The listing builds one solid part. Answer for the finished solid, in the listing's coordinates (mm). A direction names the side the tool comes from. Round coordinates to 2 decimals unless told otherwise and drop trailing zeros. Loops run counter-clockwise (first coordinate to the right, second up) from the corner with the lowest first, then second, coordinate; pieces in that order, holes last. Notation, with made-up numbers: M 67,-18.5 L 104,-18.5 A11 ccw 104,-10.5 Z; hole C 70.25,31.25 d8. An arc over 180 degrees is marked long. Answer as a JSON object with one key per item and string values.
```python
from build123d import *

# Parameters (mm, degrees)
SKETCH1_W           = 20
SKETCH1_H           = 42
BOSS_EXTRUDE1_DEPTH = 7.6
CUT_EXTRUDE1_DEPTH  = 4
THICKEN1_START      = -10
THICKEN1_DEPTH      = 20
SKETCH7_W           = 16
SKETCH7_H           = 1.6
CUT_EXTRUDE6_DEPTH  = 15


# Read off the part's stored shape, not the designer's step: Thicken1
with BuildPart() as part:
    # Sketch1 → Boss-Extrude1 (new body)
    with BuildSketch(Plane(origin=(0, 0, 0), x_dir=(1, 0, 0), z_dir=(0, 1, 0))):
        Rectangle(SKETCH1_W, SKETCH1_H)
    extrude(amount=BOSS_EXTRUDE1_DEPTH)

    # Sketch2 → Cut-Extrude1 (cut)
    with BuildSketch(Plane.XZ):
        with BuildLine():
            Line((-3.5, -17.5), (3.5, -17.5))
            Line((3.5, -17.5), (3.5, -5.5))
            ThreePointArc((3.5, -5.5), (4.085786438, -4.085786438), (5.5, -3.5))
            Line((5.5, -3.5), (8.5, -3.5))
            Line((8.5, -3.5), (8.5, 0.5))
            Line((8.5, 0.5), (5.5, 0.5))
            ThreePointArc((5.5, 0.5), (4.085786438, 1.085786438), (3.5, 2.5))
            Line((3.5, 2.5), (3.5, 17.5))
            Line((3.5, 17.5), (-3.5, 17.5))
            Line((-3.5, 17.5), (-3.5, 2.5))
            ThreePointArc((-3.5, 2.5), (-4.085786438, 1.085786438), (-5.5, 0.5))
            Line((-5.5, 0.5), (-8.5, 0.5))
            Line((-8.5, 0.5), (-8.5, -3.5))
            Line((-8.5, -3.5), (-5.5, -3.5))
            ThreePointArc((-5.5, -3.5), (-4.085786438, -4.085786438), (-3.5, -5.5))
            Line((-3.5, -5.5), (-3.5, -17.5))
        make_face()
    extrude(amount=-CUT_EXTRUDE1_DEPTH, mode=Mode.SUBTRACT)

    # Thicken1 outline → Thicken1 (add)
    with BuildSketch(Plane.YZ.offset(THICKEN1_START)):
        Polygon((0, -23), (9.6, -23), (9.6, 23), (0, 23), (0, 21), (7.6, 21), (7.6, -21), (0, -21), align=None)
    extrude(amount=THICKEN1_DEPTH)

    # Sketch7 → Cut-Extrude6 (cut)
    with BuildSketch(Plane(origin=(0, 0, -23), x_dir=(-1, 0, 0), z_dir=(0, 0, -1))):
        with Locations((0, 7.2)):
            Rectangle(SKETCH7_W, SKETCH7_H)
    extrude(amount=-CUT_EXTRUDE6_DEPTH, mode=Mode.SUBTRACT)


solid = part.part
```
Item 1: The part is cut by section C-C (z = -3). Give the vertices of the cut face in (x, y), then the cut area to 3 significant figures.
Values follow:
{"outline": "M -10,0 L -8.5,0 L -8.5,4 L 8.5,4 L 8.5,0 L 10,0 L 10,9.6 L -10,9.6 Z", "area": "124 mm^2"}
Item 2: Straight lines are drawn through the part: line 1 (Y direction, x = 2.5, z = -11); line 2 (Z direction, x = -0.25, y = 3.5); line 3 (X direction, y = 3.75, z = -12). For each, find the intervals that lie inside material, in ascending order.
Values follow:
{"line 1": "4 to 6.4, 8 to 9.6", "line 2": "-23 to -17.5, 17.5 to 23", "line 3": "-10 to -3.5, 3.5 to 10"}
Item 3: The part is cut by section A-A (z = -18.5). Give the vertices of the cut face in (x, y), then the cut area to 3 significant figures.
Values follow:
{"outline": "M -10,0 L 10,0 L 10,9.6 L -10,9.6 Z; hole M -8,6.4 L 8,6.4 L 8,8 L -8,8 Z", "area": "166 mm^2"}
Item 4: The part is cut by section D-D (z = -10). Give the vertices of the cut face in (x, y).
Values follow:
{"outline": "M -10,0 L -3.5,0 L -3.5,4 L 3.5,4 L 3.5,0 L 10,0 L 10,9.6 L -10,9.6 Z; hole M -8,6.4 L 8,6.4 L 8,8 L -8,8 Z"}
Item 5: The part is cut by section B-B (x = -6.75). Give the vertices of the cut face in (y, z), then the cut area to 3 significant figures.
Values follow:
{"outline": "M 0,-23 L 6.4,-23 L 6.4,-8 L 8,-8 L 8,-23 L 9.6,-23 L 9.6,23 L 0,23 L 0,0.5 L 4,0.5 L 4,-3.5 L 0,-3.5 Z", "area": "402 mm^2"}
Item 6: A flat-ended cylindrical pin translates along its axis: P1, Ø4, axis at x = -7, y = 7.5, coming from the -Z side. Find the tip coordinate at first contact, or state that the pin passes through.
Values follow:
{"P1": "z = -23"}
Item 7: Determine the mould class of faces 4 (the face through (-5, 0, 5)), 5 (the face through (10, 5, 0)), 6 (the face through (-8, 7, -16)) for opening direction X: released by +X, released by -X, zero draft, split by the parting line, or undercut.
Values follow:
{"face 4": "zero draft", "face 5": "released by +X", "face 6": "undercut"}
Item 8: Which of the six approach directions +Z, -Z, +X, -X, +Y, -Y give full straight-line access (tool end or side, diameter ignored) to faces 1 (the face through (0, 9.6, 0)), 2 (the face through (8, 7, -16)), 3 (the face through (-7, 2, -3.5))?
Values follow:
{"face 1": "+Z, -Z, +X, -X, +Y", "face 2": "-Z", "face 3": "-Y"}
